Can you work these out from the drawing? Everything is in mm from the part's minimum corner. Coordinates: 2 decimals unless noted, no trailing zeros. Write each loop counter-clockwise with the first axis right and the second up, starting at its lowest first coordinate (ties: lowest second). Pieces come first, ordered by that corner, then holes.
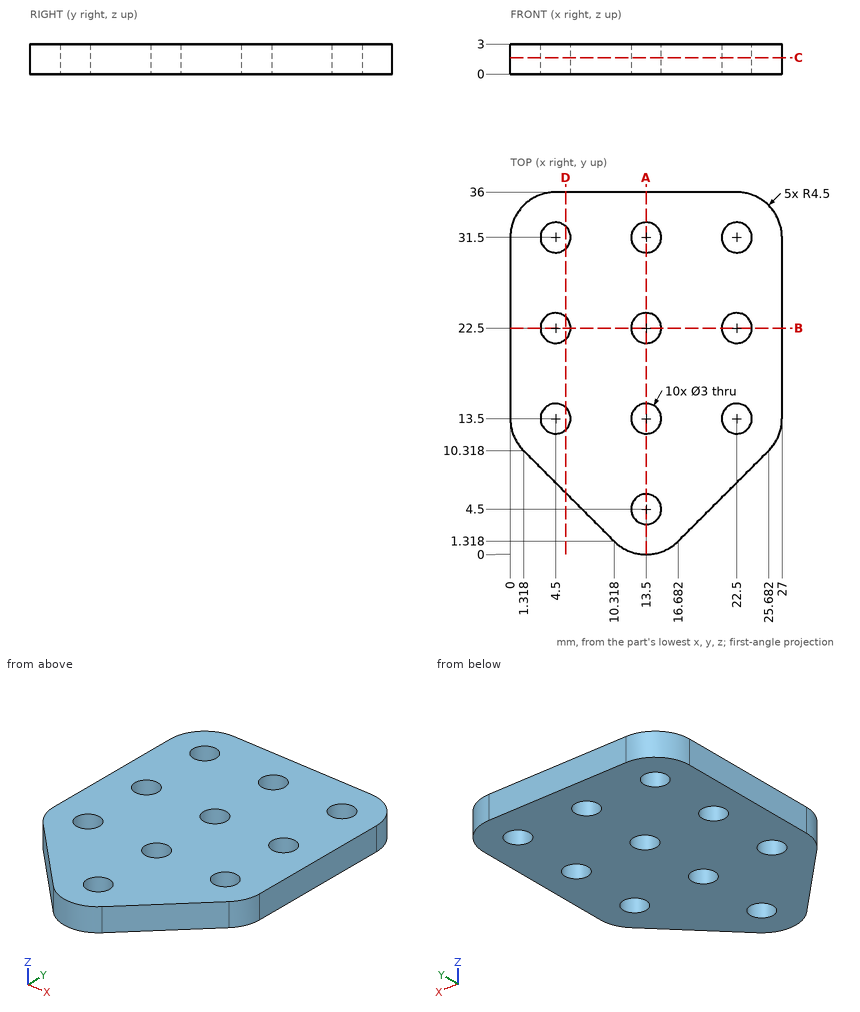
1. For pin 1 Ø5 at (x, y) = (22.5, 22.5) entering from +Z; pin 2 Ø1.8 at (x, y) = (13.5, 22.5) entering from -Z, each with a flat end and sliding along its axis, tell me the tip position at first contact or that it passes through.
2. I want a section at C-C (z = 1.65). State how many separate pieces and enclosed holes the cut face has, then the cut area to 3 significant figures.
3. I want a section at A-A (x = 13.5). List the corners of the cut face in (y, z) for me.
4. I want a section at B-B (y = 22.5). List the corners of the cut face in (x, z) for me.
5. If I drill on line 1 (X direction, y = 31.5, z = 2.35); line 2 (Y direction, x = 13.5, z = 1.55); line 3 (Y direction, x = 21.25, z = 0.95), over which ranges is the centre line in solid material (lowest first)?
6. I want a section at D-D (x = 5.5). List the corners of the cut face in (y, z) for me.
Response values:
1. pin 1: stops at z = 3
1. pin 2: passes through
2. separate pieces: 1
2. enclosed holes: 10
2. area: 755 mm2
3. outline: (0, 0) - (3, 0) - (3, 3) - (0, 3) - close; (6, 0) - (12, 0) - (12, 3) - (6, 3) - close; (15, 0) - (21, 0) - (21, 3) - (15, 3) - close; (24, 0) - (30, 0) - (30, 3) - (24, 3) - close; (33, 0) - (36, 0) - (36, 3) - (33, 3) - close
4. outline: (0, 0) - (3, 0) - (3, 3) - (0, 3) - close; (6, 0) - (12, 0) - (12, 3) - (6, 3) - close; (15, 0) - (21, 0) - (21, 3) - (15, 3) - close; (24, 0) - (27, 0) - (27, 3) - (24, 3) - close
5. line 1: x = 0 to 3, 6 to 12, 15 to 21, 24 to 27
5. line 2: y = 0 to 3, 6 to 12, 15 to 21, 24 to 30, 33 to 36
5. line 3: y = 5.89 to 12.67, 14.33 to 21.67, 23.33 to 30.67, 32.33 to 36
6. outline: (6.14, 0) - (12.38, 0) - (12.38, 3) - (6.14, 3) - close; (14.62, 0) - (21.38, 0) - (21.38, 3) - (14.62, 3) - close; (23.62, 0) - (30.38, 0) - (30.38, 3) - (23.62, 3) - close; (32.62, 0) - (36, 0) - (36, 3) - (32.62, 3) - close
